from build123d import *

# Parameters (mm, degrees)
SKETCH1_R           = 2
BOSS_EXTRUDE1_DEPTH = 1.5
BOSS_EXTRUDE2_START = -3
BOSS_EXTRUDE2_DEPTH = 20
BOSS_EXTRUDE3_DEPTH = 1
CHAMFER1_SIZE       = 1.5
FILLET1_R           = 3


with BuildPart() as part:
    # Sketch1 → Boss-Extrude1 (new, symmetric)
    with BuildSketch(Plane.XY):
        with BuildLine():
            Line((-23.993973904, -3.008018028), (-15, -14.95))
            Line((-15, -14.95), (15, -14.95))
            Line((15, -14.95), (23.993973904, -3.008018028))
            ThreePointArc((23.993973904, -3.008018028), (25, 0), (23.993973904, 3.008018028))
            Line((23.993973904, 3.008018028), (15, 14.95))
            Line((15, 14.95), (-15, 14.95))
            Line((-15, 14.95), (-23.993973904, 3.008018028))
            ThreePointArc((-23.993973904, 3.008018028), (-25, 0), (-23.993973904, -3.008018028))
        make_face()
        with Locations((-20, 0)):
            Circle(SKETCH1_R, mode=Mode.SUBTRACT)
        with Locations(Location((20, 0, 0), (0, 0, 180))):
            Circle(SKETCH1_R, mode=Mode.SUBTRACT)
        Polygon((-14.95, 3), (-7, 10.95), (7, 10.95), (14.95, 3), (14.95, -10.95), (-14.95, -10.95), align=None, mode=Mode.SUBTRACT)
    extrude(amount=BOSS_EXTRUDE1_DEPTH, both=True)

    # Sketch2 → Boss-Extrude2 (add)
    # profile 1 of 2: a face of its own
    with BuildSketch(Plane(origin=(0, 0, -1.5), x_dir=(-1, 0, 0), z_dir=(0, 0, -1)).offset(BOSS_EXTRUDE2_START)):
        Polygon((-15.95, 3.414213562), (-7.414213562, 11.95), (7.414213562, 11.95), (15.95, 3.414213562), (15.95, -11.95), (-15.95, -11.95), align=None)
        Polygon((14.95, -10.95), (-14.95, -10.95), (-14.95, 3), (-7, 10.95), (7, 10.95), (14.95, 3), align=None, mode=Mode.SUBTRACT)
    # profile 2 of 2: a face of its own
    with BuildSketch(Plane(origin=(0, 0, -1.5), x_dir=(-1, 0, 0), z_dir=(0, 0, -1)).offset(BOSS_EXTRUDE2_START)):
        Polygon((-11.25, 1.467409819), (-5.467409819, 7.25), (5.467409819, 7.25), (11.25, 1.467409819), (11.25, -7.25), (-11.25, -7.25), align=None)
    extrude(amount=BOSS_EXTRUDE2_DEPTH)


with BuildPart() as boss_extrude2_piece_1:
    # of the separate pieces the step leaves, piece 1, a body of its own (boss_extrude2_pieces)
    add(part.part.solids().sort_by_distance((11.25, 1.467409819, 1.5))[0])



with BuildPart() as boss_extrude2_piece_2:
    # of the separate pieces the step leaves, piece 2, a body of its own (boss_extrude2_pieces)
    add(part.part.solids().sort_by_distance((-23.993973904, 3.008018028, -1.5))[0])


with BuildPart() as boss_extrude2_piece_1_1:
    add(boss_extrude2_piece_1.part)

    add(boss_extrude2_piece_2.part)  # Boss-Extrude3 merges Boss-Extrude2 piece 2
    # Sketch3 → Boss-Extrude3 (add)
    with BuildSketch(Plane(origin=(0, 0, -18.5), x_dir=(-1, 0, 0), z_dir=(0, 0, -1))):
        Polygon((15.95, -11.95), (15.95, 3.414213562), (7.414213562, 11.95), (-7.414213562, 11.95), (-15.95, 3.414213562), (-15.95, -11.95), align=None)
    extrude(amount=-BOSS_EXTRUDE3_DEPTH)

    # Chamfer1
    chamfer1_edges = [boss_extrude2_piece_1_1.edges().sort_by_distance(p)[0] for p in [
        (-22, 0, 1.5),
        (22, 0, 1.5),
    ]]
    chamfer(chamfer1_edges, length=CHAMFER1_SIZE)

    # Fillet1
    fillet1_edges = [boss_extrude2_piece_1_1.edges().sort_by_distance(p)[0] for p in [
        (-5.467409819, 7.25, -8),
        (5.467409819, 7.25, -8),
        (11.25, -7.25, -8),
        (-11.25, -7.25, -8),
        (-11.25, 1.467409819, -8),
        (-15, 14.95, 0),
        (15, 14.95, 0),
        (15, -14.95, 0),
        (-15, -14.95, 0),
        (14.95, -10.95, -8),
        (14.95, 3, -8),
        (7, 10.95, -8),
        (-7, 10.95, -8),
        (-14.95, 3, -8),
        (-14.95, -10.95, -8),
    ]]
    fillet(fillet1_edges, radius=FILLET1_R)


solid = boss_extrude2_piece_1_1.part
Can you work these out from the model? Positions are in its coordinate system, mm. A direction names the side the tool comes from. Give positions to 0.01 mm unless a question says otherwise; leave off trailing zeros. Write each loop counter-clockwise with the first axis right and the second up, starting at its lowest first coordinate (ties: lowest second). Pieces come first, ordered by that corner, then holes. Notation, with made-up numbers: M -34.5,-34 L -8.5,-34 A17 cw -8.5,-22 Z; hole C 73.5,32 d2. An arc over 180 degrees is marked long. Answer in a Markdown table with one row per item. Add a question column.
Item 1: We'd pull the mould along X, two halves only. Please class faces 1 (the flat face through (0, -14.95, 0)), 2 (the cylindrical face through (14.83, -14.64, 0.02)), 3 (the flat face through (-19.89, 8.46, 0.02)), 4 (the cylindrical face through (21.6, 1.2, -0.8)): released by +X, released by -X, zero draft, split by the parting line, or undercut.
Item 2: Imagine slicing it at D-D, the plane y = -5.75. Write out the boundary of the cut face in (x, z), plus the area to 3 significant figures.
Item 3: Please list where these lines run through material, in increasing order: L1, parallel to X at y = -4, z = -12.5; L2, parallel to Y at x = 3.5, z = -3.5.
Item 4: On a 3-axis mill with a long thin cutter (end or side, diameter ignored), from which of +Z, -Z, +X, -X, +Y, -Y can I reach the whole of each face in a straight line? I mean faces 5 (the cylindrical face through (-14.86, 14.626, -0.021)), 6 (the flat face through (0, 11.95, -10)), 7 (the flat face through (0, -10.95, -8)). Say none if no direction works.
Item 5: For pin 1 Ø8 at (x, z) = (-7.5, -7) entering from +Y; pin 2 Ø5 at (x, z) = (11.5, -13.5) entering from -Y; pin 3 Ø10.5 at (y, z) = (-2.5, -12.5) entering from +X, each with a flat end and sliding along its axis, tell me the tip position at first contact or that it passes through.
Item 6: Imagine slicing it at B-B, the plane x = -20. Write out the boundary of the cut face in (y, z).
Item 7: Imagine slicing it at A-A, the plane z = -2. State how many separate pieces and enclosed holes the cut face has, plus the area to 3 significant figures.
Item 8: Imagine slicing it at C-C, the plane x = -2. Write out the boundary of the cut face in (y, z).
Evaluation:
| question | item | result |
|---|---|---|
| 1 | face 1 | zero draft |
| 1 | face 2 | released by +X |
| 1 | face 3 | released by -X |
| 1 | face 4 | undercut |
| 2 | outline | M -21.93,-1.5 L -15.95,-1.5 L -15.95,-18.5 L 15.95,-18.5 L 15.95,-1.5 L 21.93,-1.5 L 21.93,1.5 L 14.95,1.5 L 14.95,-17.5 L 10.85,-17.5 L 10.85,1.5 L -10.85,1.5 L -10.85,-17.5 L -14.95,-17.5 L -14.95,1.5 L -21.93,1.5 Z |
| 2 | area | 518 mm² |
| 3 | L1 | x = -15.95 to -14.95, -11.25 to 11.25, 14.95 to 15.95 |
| 3 | L2 | y = -11.95 to -10.95, -7.25 to 7.25, 10.95 to 11.95 |
| 4 | face 5 | +Z, -Z, -X, +Y |
| 4 | face 6 | -Z, +X, -X, +Y |
| 4 | face 7 | +Z |
| 5 | pin 1 | stops at y = 11.95 |
| 5 | pin 2 | stops at y = -11.95 |
| 5 | pin 3 | stops at x = 15.95 |
| 6 | outline | M -8.31,-1.5 L -2,-1.5 L -2,0 L -3.5,1.5 L -8.31,1.5 Z; M 2,-1.5 L 8.31,-1.5 L 8.31,1.5 L 3.5,1.5 L 2,0 Z |
| 7 | separate pieces | 2 |
| 7 | enclosed holes | 1 |
| 7 | area | 391 mm² |
| 8 | outline | M -14.95,-1.5 L -11.95,-1.5 L -11.95,-18.5 L 11.95,-18.5 L 11.95,-1.5 L 14.95,-1.5 L 14.95,1.5 L 10.95,1.5 L 10.95,-17.5 L 7.25,-17.5 L 7.25,1.5 L -7.25,1.5 L -7.25,-17.5 L -10.95,-17.5 L -10.95,1.5 L -14.95,1.5 Z |
